Autodesk Fusion 360 part; units mm, degrees
sketch "Base and Mounts" plane through (0, 0, 0) normal (0, 0, 1) x (1, 0, 0)
  line L0 (-55.5, 25) -> (55.5, 25) construction
  line L1 (55.5, 25) -> (55.5, -25) construction
  line L2 (55.5, -25) -> (-55.5, -25) construction
  line L3 (-55.5, -25) -> (-55.5, 25) construction
  line L4 (-55.5, 25) -> (55.5, -25) construction
  line L5 (55.5, 25) -> (-55.5, -25) construction
  circle A0 centre (-55.5, 25) radius 1.55
  circle A1 centre (55.5, 25) radius 1.55
  circle A2 centre (-55.5, -25) radius 1.55
  circle A3 centre (55.5, -25) radius 1.55
  line L6 (-59.55, 29.05) -> (-51.45, 29.05)
  line L7 (-51.45, 29.05) -> (-51.45, 20.95)
  line L8 (-51.45, 20.95) -> (-59.55, 20.95)
  line L9 (-59.55, 20.95) -> (-59.55, 29.05)
  line L10 (-59.55, 29.05) -> (-51.45, 20.95) construction
  line L11 (-51.45, 29.05) -> (-59.55, 20.95) construction
  line L12 (51.45, 29.05) -> (59.55, 29.05)
  line L13 (59.55, 29.05) -> (59.55, 20.95)
  line L14 (59.55, 20.95) -> (51.45, 20.95)
  line L15 (51.45, 20.95) -> (51.45, 29.05)
  line L16 (51.45, 29.05) -> (59.55, 20.95) construction
  line L17 (59.55, 29.05) -> (51.45, 20.95) construction
  line L18 (51.45, -20.95) -> (59.55, -20.95)
  line L19 (59.55, -20.95) -> (59.55, -29.05)
  line L20 (59.55, -29.05) -> (51.45, -29.05)
  line L21 (51.45, -29.05) -> (51.45, -20.95)
  line L22 (51.45, -20.95) -> (59.55, -29.05) construction
  line L23 (59.55, -20.95) -> (51.45, -29.05) construction
  line L24 (-59.55, -20.95) -> (-51.45, -20.95)
  line L25 (-51.45, -20.95) -> (-51.45, -29.05)
  line L26 (-51.45, -29.05) -> (-59.55, -29.05)
  line L27 (-59.55, -29.05) -> (-59.55, -20.95)
  line L28 (-59.55, -20.95) -> (-51.45, -29.05) construction
  line L29 (-51.45, -20.95) -> (-59.55, -29.05) construction
  line L30 (-51.45, 29.05) -> (51.45, 29.05)
  line L31 (59.55, 20.95) -> (59.55, -20.95)
  line L32 (51.45, -29.05) -> (-51.45, -29.05)
  line L33 (-59.55, -20.95) -> (-59.55, 20.95)
  point P0 (-55.5, 25)
  point P1 (55.5, 25)
  point P2 (55.5, -25)
  point P3 (-55.5, -25)
  dimension "d6" = 111
  dimension "d7" = 50
  dimension "d8" = 3.1
  dimension "d9" = 3.1
  dimension "d10" = 3.1
  dimension "d11" = 3.1
  dimension "d12" = 4.05
  dimension "d13" = 4.05
  dimension "d14" = 4.05
  dimension "d15" = 4.05
  dimension "d16" = 4.05
  dimension "d17" = 4.05
  dimension "d18" = 4.05
  dimension "d19" = 4.05
  dimension "d25" = 4.05
extrude "Extrude1" add sketch "Base and Mounts" along normal blind 10 contours L6 L7 L8 L9 | L12 L13 L14 L15 | L24 L25 L26 L27 | L18 L19 L20 L21 makes body 1 at (56.7356, 25.9359, 6.6667) makes body 2 at (55.4614, -23.4505, 6.6667) makes body 3 at (-55.5386, 26.5495, 6.6667) makes body 4 at (-54.2644, -24.0641, 6.6667)
extrude "Extrude2" add sketch "Base and Mounts" along normal blind 4 contours L7 L8 L14 L15 L18 L21 L24 L25 L30 L31 L32 L33 bodies 1 2 3 4
sketch "Cutouts" plane through (0, 0, 4) normal (0, 0, 1) x (-1, 0, 0)
  line L0 (51.45, 20.95) -> (51.45, 29.05)
  line L1 (51.45, 29.05) -> (-51.45, 29.05)
  line L2 (-51.45, 29.05) -> (-51.45, 20.95)
  line L3 (-51.45, 20.95) -> (-59.55, 20.95)
  line L4 (-59.55, 20.95) -> (-59.55, -20.95)
  line L5 (-59.55, -20.95) -> (-51.45, -20.95)
  line L6 (-51.45, -20.95) -> (-51.45, -29.05)
  line L7 (-51.45, -29.05) -> (51.45, -29.05)
  line L8 (51.45, -29.05) -> (51.45, -20.95)
  line L9 (51.45, -20.95) -> (59.55, -20.95)
  line L10 (59.55, -20.95) -> (59.55, 20.95)
  line L11 (59.55, 20.95) -> (51.45, 20.95)
  line L12 (59.55, -20.95) -> (59.549, -20.95)
  line L13 (59.549, -20.95) -> (59.549, 20.95)
  line L14 (59.549, 20.95) -> (59.55, 20.95)
  line L15 (59.55, 20.95) -> (59.55, -20.95)
  line L16 (59.549, -20.95) -> (51.449, -20.95)
  line L17 (51.449, -20.95) -> (51.449, 20.95)
  line L18 (51.449, 20.95) -> (59.549, 20.95)
  line L19 (59.549, 20.95) -> (59.549, -20.95)
  line L20 (51.449, -20.95) -> (-51.45, -20.95)
  line L21 (-51.45, -20.95) -> (-51.45, 20.95)
  line L22 (-51.45, 20.95) -> (51.449, 20.95)
  line L23 (51.449, 20.95) -> (51.449, -20.95)
  point P0 (59.55, 20.95)
  dimension "d27" = 0.001
  dimension "d28" = 8.1
  dimension "d29" = 41.9
  dimension "d30" = 8.101
  dimension "d41" = 41.9
  dimension "d42" = 41.9
extrude "Extrude3" cut sketch "Cutouts" against normal up to surface (4 mm away) contours L17 L20 L21 L22 L23 bodies 1
extrude "Extrude4" cut sketch "Cutouts" against normal up to surface (4 mm away) contours L9 L10 L11 L13 L15 L16 L17 L18 L19 L23 bodies 1
fillet "Fillet5" radius 2 4 edges at (59.55, -29.05, 5) (-59.55, -29.05, 5) (-59.55, 29.05, 5) (59.55, 29.05, 5) on bodies 1
equation "HoleSpacingX = 50 mm"
equation "HoleSpacingY = 111 mm"
equation "ThreadedInsertDiameter = 3.1 mm"
equation "ThreadedInsertHeight = 4 mm"
equation "ThreadedInsertClearance = 2.5 mm"
equation "d6 = HoleSpacingY"
equation "d7 = HoleSpacingX"
equation "d8 = ThreadedInsertDiameter"
equation "d9 = ThreadedInsertDiameter"
equation "d10 = ThreadedInsertDiameter"
equation "d11 = ThreadedInsertDiameter"
equation "d12 = ThreadedInsertClearance + ( ThreadedInsertDiameter / 2 )"
equation "d13 = d12"
equation "d14 = d12"
equation "d15 = d12"
equation "d16 = d12"
equation "d17 = d12"
equation "d18 = d12"
equation "d19 = d12"
equation "MountHeight = 6 mm"
equation "d21 = MountHeight + ThreadedInsertHeight"
equation "d23 = ThreadedInsertHeight"
equation "d25 = d12"
equation "DebugHeaderCutoutWidth = 0.001 mm"
equation "d27 = DebugHeaderCutoutWidth"
equation "d28 = 2 * d12"
equation "d29 = d42"
equation "d41 = d42"
Model file for the job. Use its own axes, mm. A direction names the side the tool comes from. Give positions to 0.01 mm unless a question says otherwise; leave off trailing zeros. Order: outer loops, then holes, each group sorted by start corner. A loop starts at its lowest first (then second) coordinate and runs counter-clockwise, first axis right, second up.
1) 3-axis set-ups, long thin cutter, end or side, ignore diameter. For faces 1 (the flat face through (55, -20.95, 7)), 2 (the flat face through (-51.45, 25, 7)), 3 (the flat face through (-5, -20.95, 3)), 4 (the cylindrical face through (58.98, 28.45, 5.07)), 5 (the flat face through (-53.8, -24.9, 10)): which of +Z, -Z, +X, -X, +Y, -Y reach the whole face in a straight line?
2) Saw through at B-B, the plane y = 25. Write the cut outline in (x, z).
3) Saw through at C-C, the plane x = -42. Write the cut outline in (y, z), then the cut area to 3 significant figures.
4) Wall check: probe 1 along Y at (x, z) = (-55.5, 4.5); probe 2 along Y at (x, z) = (55.5, 2.5); probe 3 along Y at (x, z) = (10, 2.75). Give the ranges that are in metal, low to high.
5) Pin check, flat tips, straight feed: pin 1 (1.9 mm diameter, centred on x = -55.5, y = -25, fed in from -Z); pin 2 (1.5 mm diameter, centred on y = -10, z = 4, fed in from -X); pin 3 (5 mm diameter, centred on x = 29, y = 21.5, fed in from +Z). Stop position of each tip, or through.
6) Saw through at D-D, the plane x = -55.5. Write the cut outline in (y, z).
7) Saw through at A-A, the plane z = 6.25. Write the cut outline in (x, y).
Computed:
1. face 1: +Z, +X, -X
1. face 2: +Z, +Y, -Y
1. face 3: +Z, -Z, -X
1. face 4: +Z, -Z, +X, +Y
1. face 5: +Z, +X, -X, +Y, -Y
2. outline: (-59.55, 0) - (-57.05, 0) - (-57.05, 10) - (-59.55, 10) - close; (-53.95, 0) - (53.95, 0) - (53.95, 10) - (51.45, 10) - (51.45, 4) - (-51.45, 4) - (-51.45, 10) - (-53.95, 10) - close; (57.05, 0) - (59.55, 0) - (59.55, 10) - (57.05, 10) - close
3. outline: (-29.05, 0) - (-20.95, 0) - (-20.95, 4) - (-29.05, 4) - close; (20.95, 0) - (29.05, 0) - (29.05, 4) - (20.95, 4) - close
3. area: 64.8 mm2
4. probe 1: y = -29.05 to -26.55, -23.45 to -20.95, 20.95 to 23.45, 26.55 to 29.05
4. probe 2: y = -29.05 to -26.55, -23.45 to 23.45, 26.55 to 29.05
4. probe 3: y = -29.05 to -20.95, 20.95 to 29.05
5. pin 1: passes through
5. pin 2: stops at x = 51.45
5. pin 3: stops at z = 4
6. outline: (-29.05, 0) - (-26.55, 0) - (-26.55, 10) - (-29.05, 10) - close; (-23.45, 0) - (-20.95, 0) - (-20.95, 10) - (-23.45, 10) - close; (20.95, 0) - (23.45, 0) - (23.45, 10) - (20.95, 10) - close; (26.55, 0) - (29.05, 0) - (29.05, 10) - (26.55, 10) - close
7. outline: (-59.55, -27.05) arc R2 ccw to (-57.55, -29.05) - (-51.45, -29.05) - (-51.45, -20.95) - (-59.55, -20.95) - close; (-59.55, 20.95) - (-51.45, 20.95) - (-51.45, 29.05) - (-57.55, 29.05) arc R2 ccw to (-59.55, 27.05) - close; (51.45, -29.05) - (57.55, -29.05) arc R2 ccw to (59.55, -27.05) - (59.55, -20.95) - (51.45, -20.95) - close; (51.45, 20.95) - (59.55, 20.95) - (59.55, 27.05) arc R2 ccw to (57.55, 29.05) - (51.45, 29.05) - close; hole circle Ø3.1 at (-55.5, -25); hole circle Ø3.1 at (-55.5, 25); hole circle Ø3.1 at (55.5, -25); hole circle Ø3.1 at (55.5, 25)
